Input: dimensioned drawing with shaded views. Units: mm. Origin: part minimum x, y, z. A direction names the side the tool comes from. Coordinates: 2 decimals unless noted, no trailing zeros. Loops run counter-clockwise (first coordinate to the right, second up) from the corner with the lowest first, then second, coordinate; pieces in that order, holes last. Notation, with made-up numbers: (45, 62) -> (64, 62) arc R7 cw to (64, 74) -> close; hole circle Ø2 at (21, -16). An arc over 180 degrees is marked (long way). Answer as CSV lines item,"result".
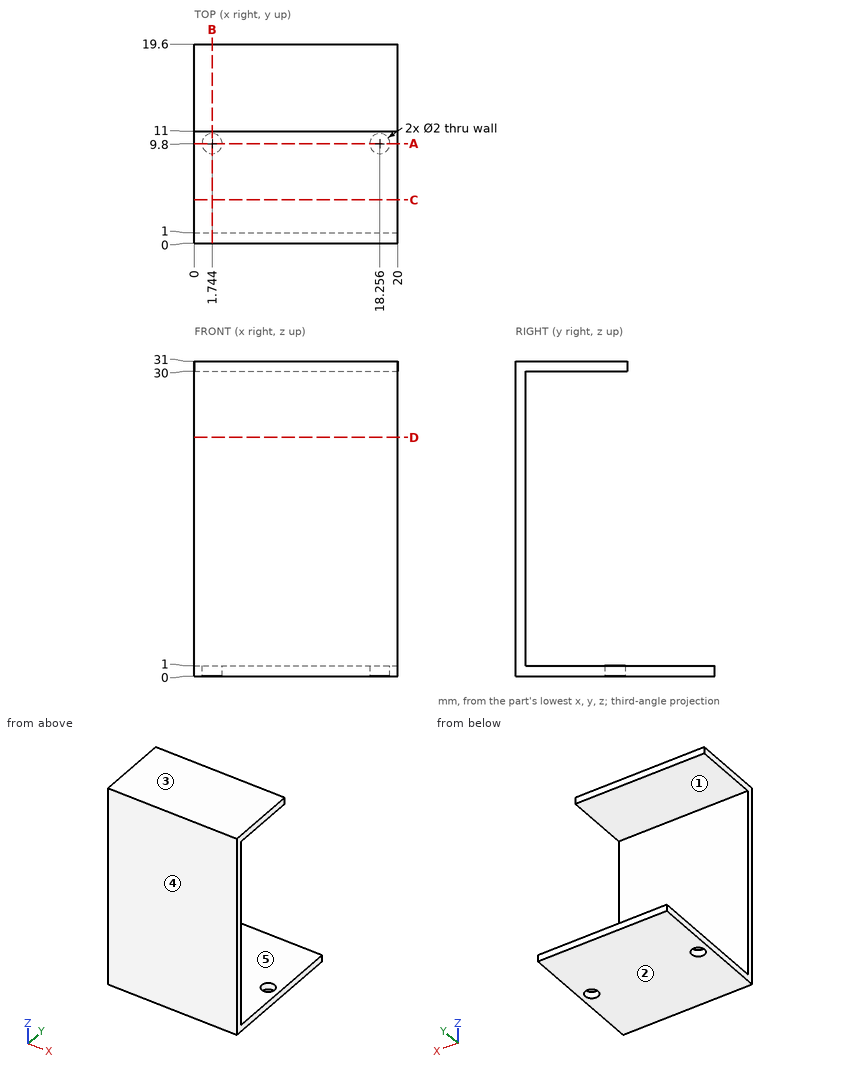
(1) Draft query along Z for the marked faces 3, 4 and 5. Return one class per face: released by +Z, released by -Z, zero draft, split by the parting line, or undercut.
Computed values:
face 3,"released by +Z"
face 4,"zero draft"
face 5,"undercut"
(2) Cut plane D-D (z = 23.5). Return the cut outline in (x, y).
Computed values:
outline,"(0, 0) -> (20, 0) -> (20, 1) -> (0, 1) -> close"
(3) Material intervals for L1, parallel to Z at x = 8.75, y = 1.25; L2, parallel to Y at x = 7.5, z = 4.5, sorted ascending. Write a range as [from, to].
Computed values:
L1,"[0, 1], [30, 31]"
L2,"[0, 1]"
(4) Cut plane A-A (y = 9.8). Return the cut outline in (x, z), then the cut area to 3 significant figures.
Computed values:
outline,"(0, 0) -> (0.74, 0) -> (0.74, 1) -> (0, 1) -> close; (0, 30) -> (20, 30) -> (20, 31) -> (0, 31) -> close; (2.74, 0) -> (17.26, 0) -> (17.26, 1) -> (2.74, 1) -> close; (19.26, 0) -> (20, 0) -> (20, 1) -> (19.26, 1) -> close"
area,"36.0 mm^2"
(5) Pin query (flat end, axial travel): pin 1 Ø2 at (x, z) = (7.5, 11.5) entering from +Y; pin 2 Ø1.8 at (x, y) = (18.256, 9.8) entering from -Z. Return the tip coordinate at first contact, or that it passes through.
Computed values:
pin 1,"y = 1"
pin 2,"z = 30"
(6) Access query for the marked faces 1 and 2. Directions: +Z, -Z, +X, -X, +Y, -Y. A direction counts if a zero-diameter tool reaches every point of the face in a straight line with its end or side. Return the directions, or none.
Computed values:
face 1,"+X, -X, +Y"
face 2,"-Z, +X, -X, +Y, -Y"
(7) Cut plane C-C (y = 4.25). Return the cut outline in (x, z).
Computed values:
outline,"(0, 0) -> (20, 0) -> (20, 1) -> (0, 1) -> close; (0, 30) -> (20, 30) -> (20, 31) -> (0, 31) -> close"
(8) Cut plane B-B (x = 1.75). Return the cut outline in (y, z), then the cut area to 3 significant figures.
Computed values:
outline,"(0, 0) -> (8.8, 0) -> (8.8, 1) -> (1, 1) -> (1, 30) -> (11, 30) -> (11, 31) -> (0, 31) -> close; (10.8, 0) -> (19.6, 0) -> (19.6, 1) -> (10.8, 1) -> close"
area,"57.6 mm^2"
